from build123d import *

# Parameters (mm, degrees)
SKETCH2_R          = 2.5
CUT_EXTRUDE1_DEPTH = 15.300349646
CHAMFER1_SIZE      = 1
CHAMFER1_SIZE2     = 0.267949192


with BuildPart() as part:
    # Sketch1 → Revolve1 (revolve)
    with BuildSketch(Plane.XY, mode=Mode.PRIVATE) as revolve1_sk:
        Polygon((0, 0), (4, 0), (4, 9.3), (3.8, 9.3), (3.8, 9.5), (5.5, 9.5), (5.5, 12), (0, 12), align=None)
    revolve(revolve1_sk.sketch.rotate(Axis((0, -5, 0), (0, 1, 0)), 90), axis=Axis((0, -5, 0), (0, 1, 0)))

    # Sketch2 → Cut-Extrude1 (cut, through all)
    with BuildSketch(Plane(origin=(0, 12, 0), x_dir=(1, 0, 0), z_dir=(0, 1, 0))):
        with Locations(Location((0, 0, 0), (0, 0, 270))):
            Circle(SKETCH2_R)
    extrude(amount=-CUT_EXTRUDE1_DEPTH, mode=Mode.SUBTRACT)

    # Chamfer1
    chamfer1_edges = [part.edges().sort_by_distance(p)[0] for p in [
        (0, 0, 4),
    ]]
    chamfer1_side = [part.faces().sort_by_distance(p)[0] for p in [
        (0, 4.65, 4),
    ]]
    chamfer(chamfer1_edges, length=CHAMFER1_SIZE, length2=CHAMFER1_SIZE2, reference=chamfer1_side[0])

    # Sketch3 → Cut-Revolve1 (revolve, cut)
    with BuildSketch(Plane.XY, mode=Mode.PRIVATE) as cut_revolve1_sk:
        Polygon((0, 12), (3.25, 12), (3.25, 11.5), (2.5, 10.200961894), (0, 10.200961894), align=None)
    revolve(cut_revolve1_sk.sketch.rotate(Axis((0, -5, 0), (0, 1, 0)), 90), axis=Axis((0, -5, 0), (0, 1, 0)), mode=Mode.SUBTRACT)


solid = part.part
Here's how the part is built. I have some questions about the finished solid (model axes, mm). A direction names the side the tool comes from. Give positions to 0.01 mm unless a question says otherwise; leave off trailing zeros. Write each loop counter-clockwise with the first axis right and the second up, starting at its lowest first coordinate (ties: lowest second). Pieces come first, ordered by that corner, then holes. Notation, with made-up numbers: (-28.5, 77) -> (24.5, 77) arc R34 cw to (24.5, 115) -> close; hole circle Ø9 at (26.25, 41). An arc over 180 degrees is marked (long way). Use one line per item in the form item = value. Start each with the question number.
1. Thinking about a two-plate mould opening in X: for faces 1 (the face through (3.905, 5.208, 0.867)), 2 (the face through (-3, 0, 0)), 3 (the face through (-2.44, 5.17, -0.54)), which applies, +X half, -X half, draft (parallel to the pull), parting line (faces both ways), or undercut?
2. Will these pins go through, and if not, where does the flat tip stop? pin 1 Ø5 at (y, z) = (2, 1.5) entering from +X; pin 2 Ø5 at (y, z) = (5, 2) entering from -X; pin 3 Ø4 at (x, z) = (2, 0) entering from +Y; pin 4 Ø6 at (x, z) = (0, 0) entering from +Y.
3. If I drill on L1, parallel to X at y = 11.8, z = 0; L2, parallel to Z at x = 2, y = 1.75; L3, parallel to Y at x = 3.5, z = -3.75, over which ranges is the centre line in solid material (lowest first)?
4. Imagine slicing it at D-D on y = 10. List the corners of the cut face in (x, z) for me, plus the area to 3 significant figures.
5. Imagine slicing it at B-B on z = 0. List the corners of the cut face in (x, y) for me.
6. Imagine slicing it at A-A on x = 0. List the corners of the cut face in (y, z) for me.
7. On a 3-axis mill with a long thin cutter (end or side, diameter ignored), from which of +Z, -Z, +X, -X, +Y, -Y can I reach the whole of each face in a straight line? I mean faces 4 (the face through (5.37, 10.77, 1.19)), 5 (the face through (1.978, 11.746, 2.579)), 6 (the face through (-1, 9.5, 4)). Say none if no direction works.
8. Imagine slicing it at C-C on y = 3. List the corners of the cut face in (x, z) for me.
Entries:
q1.face_1 = parting line
q1.face_2 = draft
q1.face_3 = undercut
q2.pin_1 = 4
q2.pin_2 = -4
q2.pin_3 = 12
q2.pin_4 = 11.07
q3.L1 = -5.5 to -3.25, 3.25 to 5.5
q3.L2 = -3.46 to -1.5, 1.5 to 3.46
q3.L3 = 9.5 to 12
q4.outline = circle Ø11 at (0, 0); hole circle Ø5 at (0, 0)
q4.area = 75.4 mm²
q5.outline = (-5.5, 9.5) -> (-3.8, 9.5) -> (-3.8, 9.3) -> (-4, 9.3) -> (-4, 1) -> (-3.73, 0) -> (-2.5, 0) -> (-2.5, 10.2) -> (-3.25, 11.5) -> (-3.25, 12) -> (-5.5, 12) -> close; (2.5, 0) -> (3.73, 0) -> (4, 1) -> (4, 9.3) -> (3.8, 9.3) -> (3.8, 9.5) -> (5.5, 9.5) -> (5.5, 12) -> (3.25, 12) -> (3.25, 11.5) -> (2.5, 10.2) -> close
q6.outline = (0, -3.73) -> (1, -4) -> (9.3, -4) -> (9.3, -3.8) -> (9.5, -3.8) -> (9.5, -5.5) -> (12, -5.5) -> (12, -3.25) -> (11.5, -3.25) -> (10.2, -2.5) -> (0, -2.5) -> close; (0, 2.5) -> (10.2, 2.5) -> (11.5, 3.25) -> (12, 3.25) -> (12, 5.5) -> (9.5, 5.5) -> (9.5, 3.8) -> (9.3, 3.8) -> (9.3, 4) -> (1, 4) -> (0, 3.73) -> close
q7.face_4 = +Y, -Y
q7.face_5 = +Y
q7.face_6 = none
q8.outline = circle Ø8 at (0, 0); hole circle Ø5 at (0, 0)
